Geometry check sheet. Reference: the model listing, model coordinates, mm. A direction names the side the tool comes from. Coordinates: 2 decimals unless noted, no trailing zeros. One line per item, written item: value. Start each with the question number.
1) Thickness scan on L1, parallel to Z at x = 40, y = -7.75; L2, parallel to Z at x = 54, y = -9.5; L3, parallel to Y at x = 79, z = -61. Record the ranges inside material, lowest first. Write a range as from..to.
2) Draft check along X on faces 1 (the cylindrical face through (28.38, -1.6, 90.92)), 2 (the cylindrical face through (33.81, -7.97, 83.39)), 3 (the cylindrical face through (104.985, -7.972, 1.796)), 4 (the flat face through (104, -6, 7)). Enter one of: pulls with the +X half, pulls with the -X half, needs draft (parallel to the pull), parting line crosses it, or undercut.
3) Sectioned sample at A-A, the plane x = 47. State how many separate pieces and enclosed holes the cut face has, then the cut area to 3 significant figures.
4) Go/stop test with flat-tipped pins: P1, Ø5, axis at x = 43.5, y = -7, coming from the +Z side; P2, Ø4, axis at y = -8, z = -66, coming from the -X side; P3, Ø2, axis at x = 42.5, y = -8.5, coming from the +Z side. Record where each tip stops, or that it passes through.
5) Access from +Z, -Z, +X, -X, +Y, -Y to the whole of each face (thin tool, end or side, straight path). Record for faces 5 (the cylindrical face through (86.52, -7.97, -17.39)), 6 (the cylindrical face through (84.988, -8.028, 1.454)).
```python
from build123d import *

# Parameters (mm, degrees)
REVOLVE_1_ANGLE     = 140
SKETCH_3_W          = 20
SKETCH_3_H          = 9
EXTRUDE_1_DEPTH     = 5
SKETCH_4_W          = 20
SKETCH_4_H          = 9
EXTRUDE_2_DEPTH     = 5
CUT_EXTRUDE_1_DEPTH = 5
FILLET_1_R          = 2
EXTRUDE_START       = -4
EXTRUDE_3_DEPTH     = 4


with BuildPart() as part:
    # 草图2 → 旋转1 (revolve, symmetric)
    with BuildSketch(Plane.XY) as revolve_1_sk:
        with BuildLine():
            ThreePointArc((102.236067977, -6), (100, -7), (97.763932023, -6))
            Line((97.763932023, -6), (85, -6))
            Line((85, -6), (85, -10))
            Line((85, -10), (105, -10))
            Line((105, -10), (105, -6))
            Line((105, -6), (102.236067977, -6))
        make_face()
    revolve(axis=Axis((0, 24.366902053, 0), (0, -1, 0)), revolution_arc=REVOLVE_1_ANGLE / 2)
    revolve(revolve_1_sk.sketch, axis=Axis((0, 24.366902053, 0), (0, 1, 0)), revolution_arc=REVOLVE_1_ANGLE / 2)

    # 草图3 → 凸台-拉伸1 (add)
    with BuildSketch(Plane(origin=(0, 0, 0), x_dir=(0.34202014332566616, 0, 0.9396926207859094), z_dir=(-0.9396926207859093, 0, 0.3420201433256661))):
        with Locations((95, -5.5)):
            Rectangle(SKETCH_3_W, SKETCH_3_H)
    extrude(amount=EXTRUDE_1_DEPTH)

    # 草图4 → 凸台-拉伸2 (add)
    with BuildSketch(Plane(origin=(0, 0, 0), x_dir=(-0.34202014332566616, 0, 0.9396926207859094), z_dir=(-0.9396926207859094, 0, -0.34202014332566616))):
        with Locations((-95, -5.5)):
            Rectangle(SKETCH_4_W, SKETCH_4_H)
    extrude(amount=EXTRUDE_2_DEPTH)

    # 草图5 → 切除-拉伸1 (cut)
    with BuildSketch(Plane(origin=(0, -6, 0), x_dir=(1, 0, 0), z_dir=(0, 1, 0))):
        with BuildLine():
            ThreePointArc((34.743766956, 81.122950869), (88.25, -6.1e-08), (34.743766843, -81.122950917))
            ThreePointArc((34.743766843, -81.122950917), (33.82406612, -83.420591403), (36.121706789, -84.340291668))
            ThreePointArc((36.121706789, -84.340291668), (91.75, 4e-08), (36.121706715, 84.3402917))
            ThreePointArc((36.121706715, 84.3402917), (33.82406608, 83.42059131), (34.743766956, 81.122950869))
        make_face()
    extrude(amount=-CUT_EXTRUDE_1_DEPTH, mode=Mode.SUBTRACT)

    # 圆角1
    fillet_1_edges = [part.edges().sort_by_distance(p)[0] for p in [
        (24.373249079, -5.5, 81.583973483),
        (31.213651945, -5.5, 100.377825899),
        (27.793450512, -1, 90.980899691),
        (27.793450512, -10, 90.980899691),
        (31.213651945, -5.5, -100.377825899),
        (24.373249079, -5.5, -81.583973483),
        (27.793450512, -1, -90.980899691),
        (27.793450512, -10, -90.980899691),
    ]]
    fillet(fillet_1_edges, radius=FILLET_1_R)

    # 草图6 → 凸台-拉伸3 (add)
    with BuildSketch(Plane.XZ.offset(10).offset(EXTRUDE_START)):
        with BuildLine():
            ThreePointArc((59.050776011, 65.582530848), (62.40217344, 62.40217344), (65.582530848, 59.050776011))
            Line((65.582530848, 59.050776011), (68.183537738, 61.392733133))
            ThreePointArc((68.183537738, 61.392733133), (64.877047174, 64.877047174), (61.392733133, 68.183537738))
            Line((61.392733133, 68.183537738), (59.050776011, 65.582530848))
        make_face()
        with BuildLine():
            ThreePointArc((79.653151344, 37.992604293), (81.532368744, 33.771812906), (83.188111589, 29.458455327))
            Line((83.188111589, 29.458455327), (86.487356808, 30.626779335))
            ThreePointArc((86.487356808, 30.626779335), (84.765947108, 35.111204919), (82.812199839, 39.499393132))
            Line((82.812199839, 39.499393132), (79.653151344, 37.992604293))
        make_face()
        with BuildLine():
            Line((91.624259814, 4.801823985), (88.129056442, 4.618648138))
            ThreePointArc((88.129056442, 4.618648138), (88.219758929, 2.310115688), (88.25, 0))
            ThreePointArc((88.25, 0), (88.219758929, -2.310115688), (88.129056442, -4.618648138))
            Line((88.129056442, -4.618648138), (91.624259814, -4.801823985))
            ThreePointArc((91.624259814, -4.801823985), (91.718559567, -2.401735007), (91.75, 0))
            ThreePointArc((91.75, 0), (91.718559567, 2.401735007), (91.624259814, 4.801823985))
        make_face()
        with BuildLine():
            ThreePointArc((83.188111589, -29.458455327), (81.532368744, -33.771812906), (79.653151344, -37.992604293))
            Line((79.653151344, -37.992604293), (82.812199839, -39.499393132))
            ThreePointArc((82.812199839, -39.499393132), (84.765947108, -35.111204919), (86.487356808, -30.626779335))
            Line((86.487356808, -30.626779335), (83.188111589, -29.458455327))
        make_face()
        with BuildLine():
            ThreePointArc((65.582530848, -59.050776011), (62.40217344, -62.40217344), (59.050776011, -65.582530848))
            Line((59.050776011, -65.582530848), (61.392733133, -68.183537738))
            ThreePointArc((61.392733133, -68.183537738), (64.877047174, -64.877047174), (68.183537738, -61.392733133))
            Line((68.183537738, -61.392733133), (65.582530848, -59.050776011))
        make_face()
    extrude(amount=EXTRUDE_3_DEPTH)


solid = part.part
```
Final values:
1. L1: z = -97.08..-82.57, -78.66..-75, 75..78.66, 82.57..97.08
1. L2: z = -90.05..-74.18, -69.8..-65.64, 65.64..69.8, 74.18..90.05
1. L3: y = -10..-6.99
2. face 1: pulls with the -X half
2. face 2: undercut
2. face 3: pulls with the +X half
2. face 4: needs draft
3. separate pieces: 4
3. enclosed holes: 0
3. area: 145 mm^2
4. P1: stops at z = 96.66
4. P2: stops at x = 51
4. P3: stops at z = 96.45
5. face 5: +Y, -Y
5. face 6: -X, +Y, -Y
